from build123d import *

# Parameters (mm, degrees)
SKETCH1_W           = 25.4
SKETCH1_H           = 25.4
SKETCH1_W_2         = 19.05
SKETCH1_H_2         = 19.05
BOSS_EXTRUDE1_DEPTH = 266.7
CUT_EXTRUDE1_DEPTH  = 270.108175275
SKETCH3_R           = 4.7625
CUT_EXTRUDE2_DEPTH  = 270.108175275


with BuildPart() as part:
    # Sketch1 → Boss-Extrude1 (new body)
    with BuildSketch(Plane.XY):
        with Locations((12.7, 12.7)):
            Rectangle(SKETCH1_W, SKETCH1_H)
        with Locations((12.7, 12.7)):
            Rectangle(SKETCH1_W_2, SKETCH1_H_2, mode=Mode.SUBTRACT)
    extrude(amount=BOSS_EXTRUDE1_DEPTH)

    # Sketch2 → Cut-Extrude1 (cut, through all)
    with BuildSketch(Plane(origin=(0, 25.4, 0), x_dir=(1, 0, 0), z_dir=(0, 1, 0))):
        Polygon((28.218627474, 4.252994852), (-38.643180904, -78.477766606), (-121.852589488, 10.228955552), (-14.467388396, 75.01098645), align=None)
    extrude(amount=-CUT_EXTRUDE1_DEPTH, mode=Mode.SUBTRACT)

    # Sketch3 → Cut-Extrude2 (cut, through all)
    with BuildSketch(Plane(origin=(0, 25.4, 0), x_dir=(1, 0, 0), z_dir=(0, 1, 0))):
        with Locations(Location((12.7, -254, 0), (0, 0, 270))):
            Circle(SKETCH3_R)
    extrude(amount=-CUT_EXTRUDE2_DEPTH, mode=Mode.SUBTRACT)


solid = part.part
Model file for the job. Use its own axes, mm. A direction names the side the tool comes from. Coordinates: 2 decimals unless noted, no trailing zeros. Order: outer loops, then holes, each group sorted by start corner. A loop starts at its lowest first (then second) coordinate and runs counter-clockwise, first axis right, second up. Notation, with made-up numbers: (45.5, 58) -> (94.5, 58) arc R12 ccw to (94.5, 70) -> close; hole circle Ø9 at (17.5, 59.5). An arc over 180 degrees is marked (long way). Return JSON: item names as keys, results as strings. Group by question number.
Item 1: Pull direction Z, two halves, no side cores. Call faces 1 (the flat face through (12.56, 1.59, 15.12)), 2 (the flat face through (13, 0, 131)), 3 (the cylindrical face through (12.909, 23.835, 249.242)), 4 (the cylindrical face through (12.909, 1.61, 249.242)): pulls with the +Z half, pulls with the -Z half, needs draft (parallel to the pull), parting line crosses it, or undercut.
Item 2: Saw through at C-C on y = 14.5. Write the cut outline in (x, z) (3 decimals), then the cut area to 3 significant figures.
Item 3: Saw through at A-A on z = 254. Write the cut outline in (x, y) (1 decimal), then the cut area to 3 significant figures.
Item 4: Saw through at D-D on z = 194.5. Write the cut outline in (x, y) (3 decimals), then the cut area to 3 significant figures.
Item 5: Tool access for faces 5 (the flat face through (0, 13, 147)), 6 (the flat face through (3.175, 13, 145)): list every direction of +Z, -Z, +X, -X, +Y, -Y with a clear straight run to the whole face (end or side of a thin tool).
Item 6: Flat gauge pin, fed straight in: P1, Ø5.5, axis at x = 12.7, z = 254, coming from the +Y side. Where does the tip first touch, or does it go through?
Item 7: Wall check: line 1 along X through (y, z) = (11.25, 32.5) (3 decimals); line 2 along X through (y, z) = (2.15, 254). Give the ranges that are in metal, low to high. Write a range as [from, to].
Item 8: Saw through at B-B on x = 12.7. Write the cut outline in (y, z) (1 decimal).
Values found:
{
 "1": {"face 1": "pulls with the -Z half", "face 2": "needs draft", "face 3": "undercut", "face 4": "undercut"},
 "2": {"outline": "(0, 30.663) -> (3.175, 26.734) -> (3.175, 266.7) -> (0, 266.7) -> close; (22.225, 3.163) -> (24.781, 0) -> (25.4, 0) -> (25.4, 266.7) -> (22.225, 266.7) -> close", "area": "1,600 mm2"},
 "3": {"outline": "(0, 0) -> (7.9, 0) -> (7.9, 3.2) -> (3.2, 3.2) -> (3.2, 22.2) -> (7.9, 22.2) -> (7.9, 25.4) -> (0, 25.4) -> close; (17.5, 0) -> (25.4, 0) -> (25.4, 25.4) -> (17.5, 25.4) -> (17.5, 22.2) -> (22.2, 22.2) -> (22.2, 3.2) -> (17.5, 3.2) -> close", "area": "222 mm2"},
 "4": {"outline": "(0, 0) -> (25.4, 0) -> (25.4, 25.4) -> (0, 25.4) -> close; hole (3.175, 3.175) -> (22.225, 3.175) -> (22.225, 22.225) -> (3.175, 22.225) -> close", "area": "282 mm2"},
 "5": {"face 5": "+Z, -Z, -X, +Y, -Y", "face 6": "+Z, -Z"},
 "6": {"P1": "passes through"},
 "7": {"line 1": "x = [0, 3.175], [22.225, 25.4]", "line 2": "x = [0, 7.94], [17.46, 25.4]"},
 "8": {"outline": "(0, 14.9) -> (3.2, 14.9) -> (3.2, 249.2) -> (0, 249.2) -> close; (0, 258.8) -> (3.2, 258.8) -> (3.2, 266.7) -> (0, 266.7) -> close; (22.2, 14.9) -> (25.4, 14.9) -> (25.4, 249.2) -> (22.2, 249.2) -> close; (22.2, 258.8) -> (25.4, 258.8) -> (25.4, 266.7) -> (22.2, 266.7) -> close"}
}
